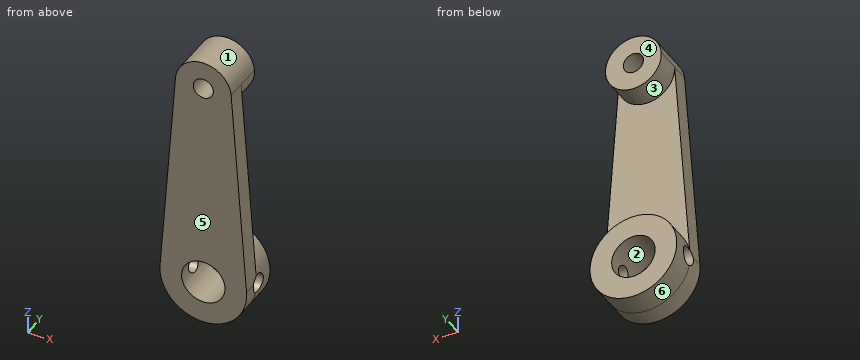
Autodesk Inventor part; units mm, degrees
ref_plane "Arbeitsebene1" through (-7, 0, 0) normal (1, 0, 0) x (0, 1, 0)
ref_plane "XZ Plane" through (0, 0, 0) normal (0, 1, 0) x (-1, 0, 0)
ref_plane "XY Plane" through (0, 0, 0) normal (0, 0, 1) x (1, 0, 0)
sketch "Skizze1" plane through (0, 0, 0) normal (0, 1, 0) x (-1, 0, 0)
  arc A0 (4.4878, 34.3309) -> (-4.4878, 34.3309) centre (0, 34) ccw
  arc A1 (-6.9811, 0.5147) -> (6.9811, 0.5147) centre (0, 0) ccw
  line L0 (4.4878, 34.3309) -> (6.9811, 0.5147)
  line L1 (-4.4878, 34.3309) -> (-6.9811, 0.5147)
  line L2 (0, 34) -> (0, 0) construction
  dimension "d0" = 34
  dimension "d1" = 14
  dimension "d2" = 9
extrude "Extrusion1" add sketch "Skizze1" along normal blind 3
sketch "Skizze2" plane through (0, 3, 0) normal (0, 1, 0) x (1, 0, 0)
  circle A0 centre (0, -34) radius 4.5
  arc A1 (-4.4878, -34.3309) -> (4.4878, -34.3309) centre (0, -34) ccw
  circle A2 centre (0, 0) radius 7
  arc A3 (6.9811, -0.5147) -> (-6.9811, -0.5147) centre (0, 0) ccw
  dimension "d5" = 9
  dimension "d6" = 14
extrude "Extrusion2" add sketch "Skizze2" along normal blind 4
sketch "Skizze3" plane through (0, 7, 34) normal (0, 1, 0) x (1, 0, 0)
  circle A0 centre (0, 0) radius 4.5
  point P0 (0, 34)
hole "Bohrung1" at (0, 7, 34) direction (0, -1, 0) diameter 3.242 depth 7
hole "Bohrung2" at (0, 7, 0) direction (0, -1, 0) diameter 7 depth 7
ref_plane "Arbeitsebene1" through (-7, 0, 0) normal (1, 0, 0) x (0, 1, 0)
sketch "Skizze4" plane through (-7, 0, 0) normal (1, 0, 0) x (0, 1, 0)
  line L0 (0, 0.5147) -> (0, 34.3309)
  line L1 (0, -7) -> (7, -7)
  point P0 (0, 0)
  point P1 (3.5, 0)
  dimension "d24" = 3.5
hole "Bohrung3" at (-7, 3.5, 0) direction (1, 0, 0) diameter 3 end through all
properties part number "2072"
Model file for the job. Use its own axes, mm. Face numbers are marked on the shaded views. A direction names the side the tool comes from. Coordinates: 2 decimals unless noted, no trailing zeros. Write each loop counter-clockwise with the first axis right and the second up, starting at its lowest first coordinate (ties: lowest second). Pieces come first, ordered by that corner, then holes. Notation, with made-up numbers: (58.5, 34.25) - (81.5, 34.25) arc R13 cw to (81.5, 41.25) - close; hole circle Ø6 at (-22.5, 81). An arc over 180 degrees is marked (long way). One line per item, written item: value. Start each with the question number.
1. Flat gauge pins, fed straight in: pin 1 (8 mm diameter, centred on x = 0, z = 0, fed in from +Y); pin 2 (7 mm diameter, centred on x = 1.5, z = 23.5, fed in from +Y); pin 3 (1 mm diameter, centred on x = -4, y = 0.5, fed in from +Z); pin 4 (1 mm diameter, centred on y = 1.5, z = 3.5, fed in from +X). Where does each tip first touch, or does it go through?
2. Slice it at B-B (x = -2.5). Write the cut outline in (y, z), plus the area to 3 significant figures.
3. Mould opens along Z. For the marked faces 1, 2, 3 and 4 say: released by +Z, released by -Z, zero draft, split by the parting line, or undercut.
4. Slice it at D-D (z = 7.5). Write the cut outline in (x, y).
5. Slice it at A-A (y = 3.5). Write the cut outline in (x, z), plus the area to 3 significant figures.
6. Tool access for the marked faces 5 and 6: list every direction of +Z, -Z, +X, -X, +Y, -Y with a clear straight run to the whole face (end or side of a thin tool).
7. Slice it at C-C (z = 28). Write the cut outline in (x, y), plus the area to 3 significant figures.
8. Probe line 1 (Y direction, x = -5.1, z = 0); line 2 (X direction, y = 5.5, z = 0); line 3 (Z direction, x = 3, y = 3.75). List the from-to ranges inside material, lowest first. Write a range as from..to.
Answers below:
1. pin 1: stops at y = 7
1. pin 2: stops at y = 3
1. pin 3: stops at z = 36.83
1. pin 4: stops at x = 6.8
2. outline: (0, -6.54) - (7, -6.54) - (7, -2.45) - (0, -2.45) - close; (0, 2.45) - (7, 2.45) - (7, 6.54) - (3, 6.54) - (3, 30.26) - (7, 30.26) - (7, 37.74) - (0, 37.74) - close
2. area: 181 mm^2
3. face 1: released by +Z
3. face 2: undercut
3. face 3: undercut
3. face 4: zero draft
4. outline: (-6.47, 0) - (6.47, 0) - (6.47, 3) - (-6.47, 3) - close
5. outline: (-6.84, -1.5) arc R7 ccw to (6.84, -1.5) - (3.16, -1.5) arc R3.5 cw to (-3.16, -1.5) - close; (-6.84, 1.5) - (-3.16, 1.5) arc R3.5 cw to (3.16, 1.5) - (6.84, 1.5) arc R7 ccw to start; circle Ø9 at (0, 34); hole circle Ø3.24 at (0, 34)
5. area: 149 mm^2
6. face 5: +Z, -Z, +X, -X, -Y
6. face 6: +Y
7. outline: (-4.95, 0) - (4.95, 0) - (4.95, 3) - (-4.95, 3) - close
7. area: 29.7 mm^2
8. line 1: y = 0..2, 5..7
8. line 2: x = -7..-3.5, 3.5..7
8. line 3: z = -6.32..-1.8, 1.8..6.32, 30.65..37.35
